Read the model definition and answer for the solid it produces. Units are mm, in the model's axes. A direction names the side the tool comes from. Coordinates: 2 decimals unless noted, no trailing zeros. Loops run counter-clockwise (first coordinate to the right, second up) from the corner with the lowest first, then second, coordinate; pieces in that order, holes last. Notation, with made-up numbers: M 43,-40 L 100,-40 A17 cw 100,-32 Z; hole C 79.5,20 d5. An arc over 180 degrees is marked long. Put each result on its own line as item: value.
from build123d import *

# Parameters (mm, degrees)
SKETCH1_R      = 2.921
EXTRUDE1_DEPTH = 44.45
SKETCH2_R      = 8.255
EXTRUDE2_DEPTH = 6.35
SKETCH3_R      = 12.827
EXTRUDE3_DEPTH = 8.89
EXTRUDE6_DEPTH = 8.89
EXTRUDE7_DEPTH = 8.89
FILLET1_R      = 1.27


with BuildPart() as part:
    # Sketch1 → Extrude1 (new body)
    with BuildSketch(Plane.XY):
        Circle(SKETCH1_R)
    extrude(amount=EXTRUDE1_DEPTH)

    # Sketch2 → Extrude2 (add)
    with BuildSketch(Plane.XY.offset(44.45)):
        Circle(SKETCH2_R)
    extrude(amount=EXTRUDE2_DEPTH)

    # Sketch3 → Extrude3 (add)
    with BuildSketch(Plane.XY.offset(50.8)):
        Circle(SKETCH3_R)
    extrude(amount=EXTRUDE3_DEPTH)

    # Sketch4 → Extrude6 (add)
    with BuildSketch(Plane.XY.offset(59.69)):
        with BuildLine():
            Line((9.631908705, 8.47102495), (14.73605764, 10.129463471))
            Line((14.73605764, 10.129463471), (17.875670303, 0.466729266))
            Line((17.875670303, 0.466729266), (12.771521368, -1.191709256))
            ThreePointArc((12.771521368, -1.191709256), (12.199201935, 3.963760987), (9.631908705, 8.47102495))
        make_face()
        with BuildLine():
            Line((-5.08, 11.778180207), (-5.08, 17.145))
            Line((-5.08, 17.145), (5.08, 17.145))
            Line((5.08, 17.145), (5.08, 11.778180207))
            ThreePointArc((5.08, 11.778180207), (0, 12.827), (-5.08, 11.778180207))
        make_face()
        with BuildLine():
            Line((11.032846956, -6.542798869), (14.187384482, -10.884647287))
            Line((14.187384482, -10.884647287), (5.967771819, -16.85654545))
            Line((5.967771819, -16.85654545), (2.813234293, -12.514697032))
            ThreePointArc((2.813234293, -12.514697032), (7.539521431, -10.377260987), (11.032846956, -6.542798869))
        make_face()
        with BuildLine():
            Line((-2.813234293, -12.514697032), (-5.967771819, -16.85654545))
            Line((-5.967771819, -16.85654545), (-14.187384482, -10.884647287))
            Line((-14.187384482, -10.884647287), (-11.032846956, -6.542798869))
            ThreePointArc((-11.032846956, -6.542798869), (-7.539521431, -10.377260987), (-2.813234293, -12.514697032))
        make_face()
        with BuildLine():
            Line((-12.771521368, -1.191709256), (-17.875670303, 0.466729266))
            Line((-17.875670303, 0.466729266), (-14.73605764, 10.129463471))
            Line((-14.73605764, 10.129463471), (-9.631908705, 8.47102495))
            ThreePointArc((-9.631908705, 8.47102495), (-12.199201935, 3.963760987), (-12.771521368, -1.191709256))
        make_face()
    extrude(amount=-EXTRUDE6_DEPTH)

    # Sketch7 → Extrude7 (add)
    with BuildSketch(Plane.XY.offset(59.69)):
        with BuildLine():
            Line((5.08, 17.145), (-5.08, 17.145))
            ThreePointArc((-5.08, 17.145), (0, 17.989354528), (5.08, 17.145))
        make_face()
    extrude(amount=-EXTRUDE7_DEPTH)

    # Fillet1
    fillet1_edges = [part.edges().sort_by_distance(p)[0] for p in [
        (-7.539521431, 10.377260987, 59.69),
        (-7.539521431, 10.377260987, 50.8),
        (5.08, 14.461590104, 59.69),
        (-5.08, 14.461590104, 59.69),
        (5.08, 14.461590104, 50.8),
        (-5.08, 14.461590104, 50.8),
        (7.539521431, 10.377260987, 59.69),
        (7.539521431, 10.377260987, 50.8),
        (15.323595836, -0.362489995, 59.69),
        (16.305863972, 5.298096369, 59.69),
        (12.183983173, 9.300244211, 59.69),
        (15.323595836, -0.362489995, 50.8),
        (12.183983173, 9.300244211, 50.8),
        (16.305863972, 5.298096369, 50.8),
        (12.199201935, -3.963760987, 59.69),
        (12.199201935, -3.963760987, 50.8),
        (4.390503056, -14.685621241, 59.69),
        (10.077578151, -13.870596369, 59.69),
        (12.610115719, -8.713723078, 59.69),
        (4.390503056, -14.685621241, 50.8),
        (12.610115719, -8.713723078, 50.8),
        (10.077578151, -13.870596369, 50.8),
        (0, -12.827, 59.69),
        (0, -12.827, 50.8),
        (-12.610115719, -8.713723078, 59.69),
        (-10.077578151, -13.870596369, 59.69),
        (-4.390503056, -14.685621241, 59.69),
        (-12.610115719, -8.713723078, 50.8),
        (-4.390503056, -14.685621241, 50.8),
        (-10.077578151, -13.870596369, 50.8),
        (-8.255, 0, 44.45),
        (-12.199201935, -3.963760987, 59.69),
        (-8.255, 0, 50.8),
        (-12.199201935, -3.963760987, 50.8),
        (-12.183983173, 9.300244211, 59.69),
        (-16.305863972, 5.298096369, 59.69),
        (-15.323595836, -0.362489995, 59.69),
        (-12.183983173, 9.300244211, 50.8),
        (-15.323595836, -0.362489995, 50.8),
        (-16.305863972, 5.298096369, 50.8),
        (0, 17.989354528, 59.69),
        (0, 17.989354528, 50.8),
    ]]
    fillet(fillet1_edges, radius=FILLET1_R)


solid = part.part
1) Find section C-C, the plane z = 8. Write down the section's boundary in (x, y), plus the area to 3 significant figures.
Answer list:
outline: C 0,0 d5.84
area: 26.8 mm^2
2) Straight lines are drawn through the part: line 1 (Z direction, x = 2, y = 13.5); line 2 (Z direction, x = -2, y = 4); line 3 (Y direction, x = 0, z = 40). For each, find the intervals that lie inside material, in ascending order. Write a range as [from, to].
Answer list:
line 1: z = [50.8, 59.69]
line 2: z = [44.45, 59.69]
line 3: y = [-2.92, 2.92]
3) Which of the six approach directions +Z, -Z, +X, -X, +Y, -Y give full straight-line access (tool end or side, diameter ignored) to faces 4 (the flat face through (4.4, -14.7, 55.3)), 5 (the cylindrical face through (-12.021, -8.552, 59.328)), 6 (the cylindrical face through (4.718, 13.984, 51.182)), 7 (the flat face through (12.15, 9.29, 55.29))?
Answer list:
face 4: +Z, -Z, -Y
face 5: +Z, -X
face 6: -Z, +X, +Y
face 7: +Z, -Z, +Y
4) Find section B-B, the plane x = 0. Write down the section's boundary in (y, z) (3 decimals).
Answer list:
outline: M -12.827,52.07 A1.27 ccw -11.557,50.8 L -9.525,50.8 A1.27 cw -8.255,49.53 L -8.255,45.72 A1.27 ccw -6.985,44.45 L -2.921,44.45 L -2.921,0 L 2.921,0 L 2.921,44.45 L 6.985,44.45 A1.27 ccw 8.255,45.72 L 8.255,49.53 A1.27 cw 9.525,50.8 L 16.719,50.8 A1.27 ccw 17.989,52.07 L 17.989,58.42 A1.27 ccw 16.719,59.69 L -11.557,59.69 A1.27 ccw -12.827,58.42 Z
5) Determine the mould class of faces 1 (the cylindrical face through (-15.92, 5.25, 51.16)), 2 (the flat face through (3, -1, 44.45)), 3 (the cylindrical face through (-4.47, -14.146, 59.328)) for opening direction X: released by +X, released by -X, zero draft, split by the parting line, or undercut.
Answer list:
face 1: released by -X
face 2: zero draft
face 3: undercut
6) Given pin 1 Ø1.5 at (y, z) = (-10.5, 51.5) entering from +X; pin 2 Ø2.5 at (y, z) = (13.5, 53.5) entering from +X; pin 3 Ø2 at (y, z) = (5, 44) entering from -X, each flat-ended and moving along its own axis, determine where each tip first touches the part or whether it passes through.
Answer list:
pin 1: stops at x = 14.19
pin 2: stops at x = 5.08
pin 3: stops at x = -6.52
7) Find section A-A, the plane z = 53.5. Write down the section's boundary in (x, y) (3 decimals).
Answer list:
outline: M -17.876,0.467 L -12.772,-1.192 A12.827 ccw -11.033,-6.543 L -14.187,-10.885 L -5.968,-16.857 L -2.813,-12.515 A12.827 ccw 2.813,-12.515 L 5.968,-16.857 L 14.187,-10.885 L 11.033,-6.543 A12.827 ccw 12.772,-1.192 L 17.876,0.467 L 14.736,10.129 L 9.632,8.471 A12.827 ccw 5.08,11.778 L 5.08,17.145 A15.704 ccw -5.08,17.145 L -5.08,11.778 A12.827 ccw -9.632,8.471 L -14.736,10.129 Z
